from build123d import *

# Parameters (mm, degrees)
SKETCH1_R           = 2.4257
BOSS_EXTRUDE1_DEPTH = 3.175
FILLET1_R           = 3.175
SKETCH2_W           = 69.85
SKETCH2_H           = 69.85
CUT_EXTRUDE1_DEPTH  = 388.727172926
FILLET3_R           = 6.35


with BuildPart() as part:
    # Sketch1 → Boss-Extrude1 (new body)
    with BuildSketch(Plane(origin=(0, 0, 0), x_dir=(1, 0, 0), z_dir=(0, 1, 0))):
        Polygon((0, 0), (203.2, 0), (203.2, 114.3), (120.65, 330.2), (0, 330.2), align=None)
        with Locations(Location((15.875, 9.525, 0), (0, 0, 270))):
            Circle(SKETCH1_R, mode=Mode.SUBTRACT)
        with Locations(Location((101.6, 9.525, 0), (0, 0, 270))):
            Circle(SKETCH1_R, mode=Mode.SUBTRACT)
        with Locations(Location((187.325, 9.525, 0), (0, 0, 270))):
            Circle(SKETCH1_R, mode=Mode.SUBTRACT)
        with Locations(Location((15.875, 104.775, 0), (0, 0, 270))):
            Circle(SKETCH1_R, mode=Mode.SUBTRACT)
        with Locations(Location((187.325, 104.775, 0), (0, 0, 270))):
            Circle(SKETCH1_R, mode=Mode.SUBTRACT)
        with Locations(Location((101.6, 104.775, 0), (0, 0, 270))):
            Circle(SKETCH1_R, mode=Mode.SUBTRACT)
        with Locations(Location((15.875, 136.525, 0), (0, 0, 270))):
            Circle(SKETCH1_R, mode=Mode.SUBTRACT)
        with Locations(Location((111.125, 136.525, 0), (0, 0, 270))):
            Circle(SKETCH1_R, mode=Mode.SUBTRACT)
        with Locations(Location((15.875, 225.425, 0), (0, 0, 270))):
            Circle(SKETCH1_R, mode=Mode.SUBTRACT)
        with Locations(Location((15.875, 314.325, 0), (0, 0, 270))):
            Circle(SKETCH1_R, mode=Mode.SUBTRACT)
        with Locations(Location((111.125, 225.425, 0), (0, 0, 270))):
            Circle(SKETCH1_R, mode=Mode.SUBTRACT)
        with Locations(Location((111.125, 314.325, 0), (0, 0, 270))):
            Circle(SKETCH1_R, mode=Mode.SUBTRACT)
    extrude(amount=BOSS_EXTRUDE1_DEPTH)

    # Fillet1
    fillet1_edges = [part.edges().sort_by_distance(p)[0] for p in [
        (0, 1.5875, -330.2),
        (120.65, 1.5875, -330.2),
        (203.2, 1.5875, -114.3),
        (203.2, 1.5875, 0),
        (0, 1.5875, 0),
    ]]
    fillet(fillet1_edges, radius=FILLET1_R)

    # Sketch2 → Cut-Extrude1 (cut, through all)
    with BuildSketch(Plane(origin=(0, 3.175, 0), x_dir=(1, 0, 0), z_dir=(0, 1, 0))):
        with Locations((63.5, 180.975)):
            Rectangle(SKETCH2_W, SKETCH2_H)
    extrude(amount=-CUT_EXTRUDE1_DEPTH, mode=Mode.SUBTRACT)

    # Fillet3
    fillet3_edges = [part.edges().sort_by_distance(p)[0] for p in [
        (98.425, 1.5875, -215.9),
        (98.425, 1.5875, -146.05),
        (28.575, 1.5875, -146.05),
        (28.575, 1.5875, -215.9),
    ]]
    fillet(fillet3_edges, radius=FILLET3_R)


solid = part.part
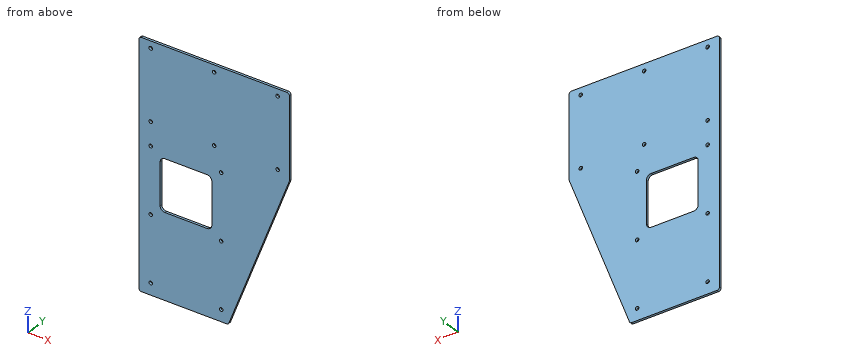
The model under review builds one solid part; all positions refer to its coordinate system, in mm. Round coordinates to 2 decimals unless told otherwise and drop trailing zeros. Write each loop counter-clockwise with the first axis right and the second up, starting at its lowest first coordinate (ties: lowest second). Pieces come first, ordered by that corner, then holes. Notation, with made-up numbers: M 58.5,56 L 86.5,56 A24 cw 86.5,94 Z; hole C -28.5,19.25 d6. An arc over 180 degrees is marked long. Use a Markdown table: item, result. Add a question column.
Q1. We need section B-B, the plane z = -193. State the section outline as (x, y) points (3 decimals).
Q2. We need section C-C, the plane y = 1.1. Count the separate pieces of the cut face and the enclosed holes in it, plus the area to 3 significant figures.
Q3. We need section A-A, the plane x = 66. State the section outline as (y, z) points (3 decimals), plus the area to 3 significant figures.
Q4. Insertion check: pin 1 (3 mm diameter, centred on x = 15.875, z = -104.775, fed in from -Y); pin 2 (1 mm diameter, centred on y = 0.5, z = -291, fed in from +X); pin 3 (1 mm diameter, centred on y = 1.5, z = -182, fed in from +X). Each pin has a flat end and moves straight along its axis. Give the tip position at first contact, or say it passes through.
Q5. To check wall thickness, follow line 1 (Z direction, x = 16.5, y = 2.9); line 2 (Z direction, x = 60.5, y = 1.3); line 3 (X direction, y = 1.9, z = -164.5) (3 decimals). State the ranges of each line that lie inside material, in increasing order.
Q6. We need section D-D, the plane x = 165. State the section outline as (y, z) points (3 decimals), plus the area to 3 significant figures.
Findings below:
| question | item | result |
|---|---|---|
| 1 | outline | M 0,0 L 28.575,0 L 28.575,3.175 L 0,3.175 Z; M 98.425,0 L 173.109,0 L 173.109,3.175 L 98.425,3.175 Z |
| 2 | separate pieces | 1 |
| 2 | enclosed holes | 13 |
| 2 | area | 53,100 mm² |
| 3 | outline | M 0,-330.2 L 3.175,-330.2 L 3.175,-215.9 L 0,-215.9 Z; M 0,-146.05 L 3.175,-146.05 L 3.175,0 L 0,0 Z |
| 3 | area | 827 mm² |
| 4 | pin 1 | passes through |
| 4 | pin 2 | stops at x = 135.83 |
| 4 | pin 3 | stops at x = 177.51 |
| 5 | line 1 | z = -330.2 to -316.67, -311.98 to -227.77, -223.08 to -138.87, -134.18 to -107.12, -102.43 to -11.87, -7.18 to 0 |
| 5 | line 2 | z = -330.2 to -215.9, -146.05 to 0 |
| 5 | line 3 | x = 0 to 28.575, 98.425 to 184.006 |
| 6 | outline | M 0,-214.208 L 3.175,-214.208 L 3.175,0 L 0,0 Z |
| 6 | area | 680 mm² |
